Check sheet for the drawn part. Datum: minimum x, y, z corner. Units: mm. A direction names the side the tool comes from. Give positions to 0.01 mm unless a question says otherwise; leave off trailing zeros. Order: outer loops, then holes, each group sorted by start corner. A loop starts at its lowest first (then second) coordinate and runs counter-clockwise, first axis right, second up. Notation, with made-up numbers: (44.5, -31) -> (72.5, -31) arc R29 cw to (72.5, 4) -> close; hole circle Ø3 at (15.25, 86). An arc over 180 degrees is marked (long way). Answer in a Markdown table with one row per item. Add a question column.
(1) Thickness scan on L1, parallel to X at y = 24.5, z = 8.25; L2, parallel to Y at x = 68, z = 9.75; L3, parallel to Z at x = 49, y = 60.5. Record the ranges inside material, lowest first. Write a range as [from, to].
(2) Set-up check for the marked faces 1 and 2: record each of +Z, -Z, +X, -X, +Y, -Y from which the full face is reachable in a straight line by a thin tool's end or side.
(3) Cross-section at D-D (y = 55). Record the cut outline in (x, z).
(4) Cross-section at A-A (z = 9.75). Record the cut outline in (x, y).
(5) Cross-section at C-C (y = 18.5). Record the cut outline in (x, z), then the cut area to 3 significant figures.
(6) Cross-section at B-B (x = 90.5). Record the cut outline in (y, z).
(7) Go/stop test with flat-tipped pins: pin 1 (2.5 mm diameter, centred on y = 54.5, z = 6.5, fed in from +X); pin 2 (2.5 mm diameter, centred on x = 61, z = 8.5, fed in from +Y); pin 3 (5 mm diameter, centred on y = 30.5, z = 9, fed in from +X); pin 4 (4.5 mm diameter, centred on x = 62, z = 4.5, fed in from +Y). Record where each tip stops, or that it passes through.
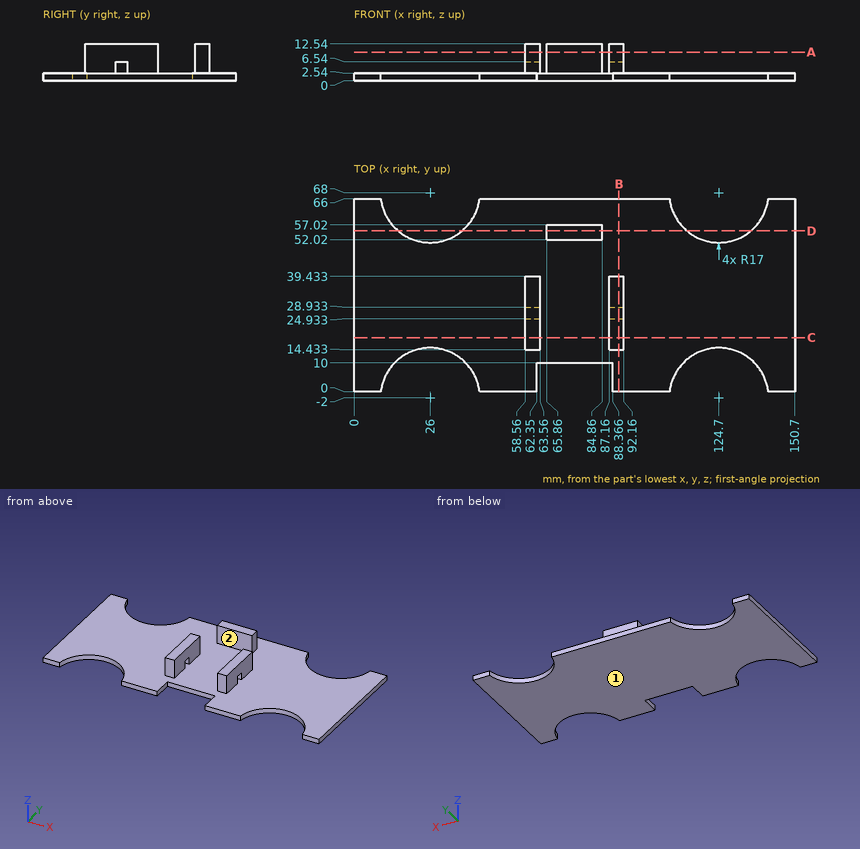
Answer below:
| question | item | result |
|---|---|---|
| 1 | L1 | x = [58.56, 63.56], [87.16, 92.16] |
| 1 | L2 | y = [52.02, 57.02] |
| 1 | L3 | z = [0, 2.54] |
| 2 | face 1 | -Z, +X, -X, +Y, -Y |
| 2 | face 2 | +Z, +X, -X, -Y |
| 3 | outline | (0, 0) -> (15.05, 0) -> (15.05, 2.54) -> (0, 2.54) -> close; (36.95, 0) -> (113.75, 0) -> (113.75, 2.54) -> (84.86, 2.54) -> (84.86, 12.54) -> (65.86, 12.54) -> (65.86, 2.54) -> (36.95, 2.54) -> close; (135.65, 0) -> (150.7, 0) -> (150.7, 2.54) -> (135.65, 2.54) -> close |
| 4 | outline | (58.56, 14.43) -> (63.56, 14.43) -> (63.56, 39.43) -> (58.56, 39.43) -> close; (65.86, 52.02) -> (84.86, 52.02) -> (84.86, 57.02) -> (65.86, 57.02) -> close; (87.16, 14.43) -> (92.16, 14.43) -> (92.16, 39.43) -> (87.16, 39.43) -> close |
| 5 | outline | (0, 0) -> (150.7, 0) -> (150.7, 2.54) -> (92.16, 2.54) -> (92.16, 12.54) -> (87.16, 12.54) -> (87.16, 2.54) -> (63.56, 2.54) -> (63.56, 12.54) -> (58.56, 12.54) -> (58.56, 2.54) -> (0, 2.54) -> close |
| 5 | area | 483 mm² |
| 6 | outline | (0, 0) -> (66, 0) -> (66, 2.54) -> (39.43, 2.54) -> (39.43, 12.54) -> (14.43, 12.54) -> (14.43, 2.54) -> (0, 2.54) -> close; hole (24.93, 2.54) -> (28.93, 2.54) -> (28.93, 6.54) -> (24.93, 6.54) -> close |
| 7 | pin 1 | stops at x = 84.86 |
| 7 | pin 2 | stops at y = 39.43 |
| 7 | pin 3 | stops at x = 92.16 |
| 7 | pin 4 | stops at y = 66 |
